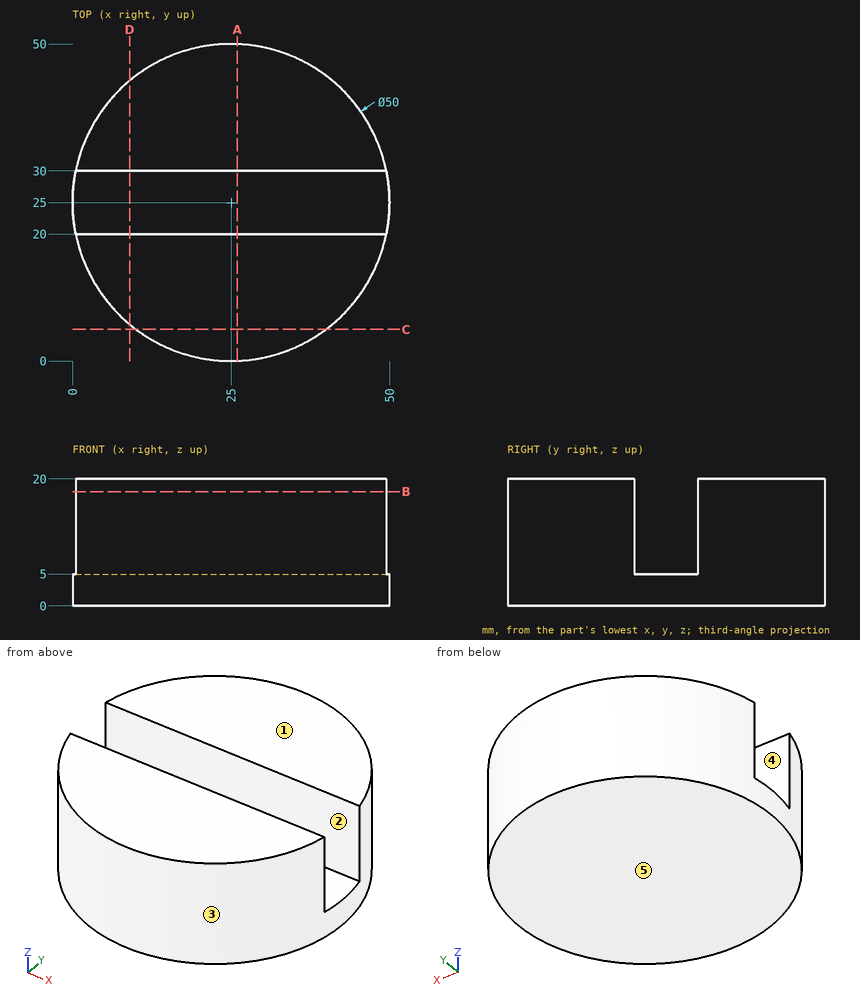
Verification items for this drawing (mm, ordinates from the low corner). A direction names the side the tool comes from. Give positions to 0.01 mm unless a question says otherwise; leave off trailing zeros. Write each loop counter-clockwise with the first axis right and the second up, starting at its lowest first coordinate (ties: lowest second). Pieces come first, ordered by that corner, then holes. Notation, with made-up numbers: (15.5, 34) -> (22.5, 34) arc R15 cw to (22.5, 56) -> close; hole circle Ø3 at (34, 80). An arc over 180 degrees is marked (long way). Use CSV: the item, a comma, the result in double quotes.
(1) Go/stop test with flat-tipped pins: pin 1 (5 mm diameter, centred on x = 23, y = 25, fed in from +Z); pin 2 (1 mm diameter, centred on y = 38.5, z = 3, fed in from +X); pin 3 (4 mm diameter, centred on y = 17.5, z = 17.5, fed in from +X). Record where each tip stops, or that it passes through.
Derived:
pin 1,"stops at z = 5"
pin 2,"stops at x = 46.35"
pin 3,"stops at x = 49.39"
(2) Sectioned sample at D-D (x = 9). Record the cut outline in (y, z).
Derived:
outline,"(5.79, 0) -> (44.21, 0) -> (44.21, 20) -> (30, 20) -> (30, 5) -> (20, 5) -> (20, 20) -> (5.79, 20) -> close"
(3) Set-up check for the marked faces 4 and 5: record each of +Z, -Z, +X, -X, +Y, -Y from which the full face is reachable in a straight line by a thin tool's end or side.
Derived:
face 4,"+Z, +X, -X"
face 5,"-Z, +X, -X, +Y, -Y"
(4) Release check for a two-part mould opening along Y. For the marked faces 1, 2 and 3 record: +Y half, -Y half, draft (parallel to the pull), parting line (faces both ways), or undercut.
Derived:
face 1,"draft"
face 2,"undercut"
face 3,"parting line"
(5) Sectioned sample at C-C (y = 5). Record the cut outline in (x, z), plus the area to 3 significant figures.
Derived:
outline,"(10, 0) -> (40, 0) -> (40, 20) -> (10, 20) -> close"
area,"600 mm^2"
(6) Sectioned sample at A-A (x = 26). Record the cut outline in (y, z), plus the area to 3 significant figures.
Derived:
outline,"(0.02, 0) -> (49.98, 0) -> (49.98, 20) -> (30, 20) -> (30, 5) -> (20, 5) -> (20, 20) -> (0.02, 20) -> close"
area,"849 mm^2"
(7) Sectioned sample at B-B (z = 18). Record the cut outline in (x, y).
Derived:
outline,"(0.51, 20) arc R25 ccw to (49.49, 20) -> close; (0.51, 30) -> (49.49, 30) arc R25 ccw to start"
(8) Material ranges on L1, parallel to Y at x = 24, z = 10.5; L2, parallel to Y at x = 11, z = 5.5; L3, parallel to X at y = 19.5, z = 11, recorded low to high.
Derived:
L1,"y = 0.02 to 20, 30 to 49.98"
L2,"y = 4.29 to 20, 30 to 45.71"
L3,"x = 0.61 to 49.39"
